Can you work these out from the model? Positions are in its coordinate system, mm. A direction names the side the tool comes from. Coordinates: 2 decimals unless noted, no trailing zeros. Order: outer loops, then holes, each group sorted by start corner. A loop starts at its lowest first (then second) coordinate and runs counter-clockwise, first axis right, second up. Notation, with made-up numbers: M -39.75,21.25 L -30.75,21.25 A17 ccw -30.75,42.25 Z; hole C -20.75,62 d10. An arc over 180 degrees is marked long. Answer as a JSON object with one key per item and string values.
from build123d import *

# Parameters (mm, degrees)
SKETCH1_W           = 67.056
SKETCH1_H           = 16.256
BOSS_EXTRUDE1_DEPTH = 6.35
SKETCH2_R           = 4.7625
BOSS_EXTRUDE2_DEPTH = 14.097
SKETCH3_R           = 2.4511
CUT_EXTRUDE1_DEPTH  = 72.964188879
CUT_EXTRUDE2_REACH  = 73.964
SKETCH4_R           = 1.0922
SKETCH6_R           = 7.3025
SKETCH6_R_2         = 4.7625
BOSS_EXTRUDE3_DEPTH = 4.572


with BuildPart() as part:
    # Sketch1 → Boss-Extrude1 (new body)
    with BuildSketch(Plane(origin=(0, 0, 0), x_dir=(1, 0, 0), z_dir=(0, 1, 0))):
        with Locations((33.528, 8.128)):
            Rectangle(SKETCH1_W, SKETCH1_H)
    extrude(amount=BOSS_EXTRUDE1_DEPTH)

    # Sketch2 → Boss-Extrude2 (add)
    with BuildSketch(Plane(origin=(0, 6.35, 0), x_dir=(1, 0, 0), z_dir=(0, 1, 0))):
        with Locations(Location((33.528, 8.128, 0), (0, 0, 90))):
            Circle(SKETCH2_R)
    extrude(amount=BOSS_EXTRUDE2_DEPTH)

    # Sketch3 → Cut-Extrude1 (cut, through all)
    with BuildSketch(Plane(origin=(0, 20.447, 0), x_dir=(1, 0, 0), z_dir=(0, 1, 0))):
        with Locations(Location((33.528, 8.128, 0), (0, 0, 270))):
            Circle(SKETCH3_R)
    extrude(amount=-CUT_EXTRUDE1_DEPTH, mode=Mode.SUBTRACT)

    # Sketch4 → Cut-Extrude2 (cut, up to next)
    with BuildSketch(Plane(origin=(0, 0, 0), x_dir=(-1, 0, 0), z_dir=(0, -1, 0)), mode=Mode.PRIVATE) as cut_extrude2_sk1:
        with Locations(Location((-25.908, 14.224, 0), (0, 0, 90))):
            Circle(SKETCH4_R)
    cut_extrude2_tool1 = extrude(cut_extrude2_sk1.sketch, amount=-CUT_EXTRUDE2_REACH, mode=Mode.PRIVATE) & part.part
    # Sketch4 → Cut-Extrude2 (cut, up to next)
    with BuildSketch(Plane(origin=(0, 0, 0), x_dir=(-1, 0, 0), z_dir=(0, -1, 0)), mode=Mode.PRIVATE) as cut_extrude2_sk2:
        with Locations(Location((-41.148, 14.224, 0), (0, 0, 90))):
            Circle(SKETCH4_R)
    cut_extrude2_tool2 = extrude(cut_extrude2_sk2.sketch, amount=-CUT_EXTRUDE2_REACH, mode=Mode.PRIVATE) & part.part
    add(cut_extrude2_tool1.solids().sort_by_distance((25.908, 0, -14.224))[0], mode=Mode.SUBTRACT)
    add(cut_extrude2_tool2.solids().sort_by_distance((41.148, 0, -14.224))[0], mode=Mode.SUBTRACT)

    # Sketch6 → Boss-Extrude3 (add)
    with BuildSketch(Plane(origin=(0, 6.35, 0), x_dir=(1, 0, 0), z_dir=(0, 1, 0))):
        with Locations(Location((33.528, 8.128, 0), (0, 0, 90))):
            Circle(SKETCH6_R)
        with Locations(Location((33.528, 8.128, 0), (0, 0, 270))):
            Circle(SKETCH6_R_2, mode=Mode.SUBTRACT)
    extrude(amount=BOSS_EXTRUDE3_DEPTH)


solid = part.part
Item 1: I want a section at B-B, the plane y = 5.5. Write out the boundary of the cut face in (x, z).
Answers follow:
{"outline": "M 0,-16.26 L 67.06,-16.26 L 67.06,0 L 0,0 Z; hole C 25.91,-14.22 d2.18; hole C 33.53,-8.13 d4.9; hole C 41.15,-14.22 d2.18"}
Item 2: I'm going to push flat-ended pins straight in: pin 1 (3 mm diameter, centred on x = 33.528, z = -8.128, fed in from -Y); pin 2 (1 mm diameter, centred on x = 21, z = -6, fed in from +Y); pin 3 (12 mm diameter, centred on x = 37.5, y = 15.5, fed in from +Z). Where does each tip first touch, or does it pass through?
Answers follow:
{"pin 1": "passes through", "pin 2": "stops at y = 6.35", "pin 3": "stops at z = -0.83"}
Item 3: Which directions (+Z, -Z, +X, -X, +Y, -Y) give clear straight access to the entire face, cutting with the end or side of a thin tool? Please do faces 4 (the flat face through (0, 3, -8)), 5 (the flat face through (35, 10.922, -13)).
Answers follow:
{"face 4": "+Z, -Z, -X, +Y, -Y", "face 5": "+Y"}
Item 4: I want a section at D-D, the plane z = -4. Write out the boundary of the cut face in (x, y), plus the area to 3 significant figures.
Answers follow:
{"outline": "M 0,0 L 67.06,0 L 67.06,6.35 L 39.55,6.35 L 39.55,10.92 L 35.9,10.92 L 35.9,20.45 L 31.15,20.45 L 31.15,10.92 L 27.5,10.92 L 27.5,6.35 L 0,6.35 Z", "area": "526 mm^2"}
Item 5: Please list where these lines run through material, in increasing order: line 1 (Y direction, x = 41, z = -11.75); line 2 (X direction, y = 5.5, z = -8); line 3 (X direction, y = 13.75, z = -6.5).
Answers follow:
{"line 1": "y = 0 to 6.35", "line 2": "x = 0 to 31.08, 35.98 to 67.06", "line 3": "x = 29.05 to 31.7, 35.36 to 38"}
Item 6: I want a section at A-A, the plane z = -8. Write out the boundary of the cut face in (x, y), plus the area to 3 significant figures.
Answers follow:
{"outline": "M 0,0 L 31.08,0 L 31.08,20.45 L 28.77,20.45 L 28.77,10.92 L 26.23,10.92 L 26.23,6.35 L 0,6.35 Z; M 35.98,0 L 67.06,0 L 67.06,6.35 L 40.83,6.35 L 40.83,10.92 L 38.29,10.92 L 38.29,20.45 L 35.98,20.45 Z", "area": "483 mm^2"}
Item 7: If we mould it in two halves opening along Z, with no side actions, what happens to faces 1 (the cylindrical face through (26.99, 3.13, -14.08)), 2 (the flat face through (33, 3, 0)), 3 (the flat face through (67.056, 3, -8))? For each: pulls with the +Z half, pulls with the -Z half, needs draft (parallel to the pull), parting line crosses it, or undercut.
Answers follow:
{"face 1": "undercut", "face 2": "pulls with the +Z half", "face 3": "needs draft"}
Item 8: I want a section at C-C, the plane x = 30. Write out the boundary of the cut face in (y, z).
Answers follow:
{"outline": "M 0,-16.26 L 6.35,-16.26 L 6.35,-14.52 L 10.92,-14.52 L 10.92,-11.33 L 20.45,-11.33 L 20.45,-4.93 L 10.92,-4.93 L 10.92,-1.73 L 6.35,-1.73 L 6.35,0 L 0,0 Z"}
